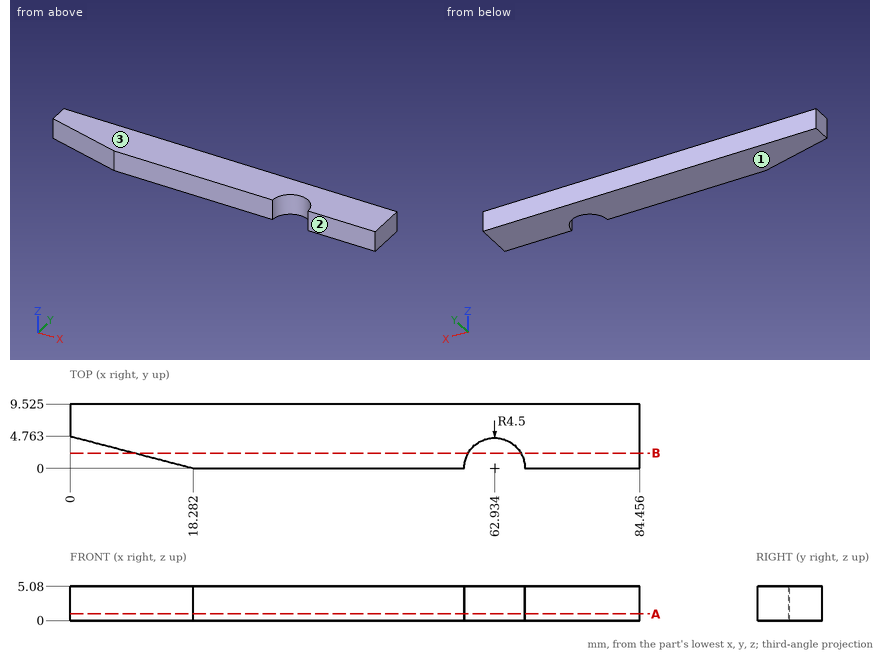
The drawing under review shows one solid part. Ordinate dimensions are in mm from its lowest x, y, z. Give positions to 0.01 mm unless a question says otherwise; leave off trailing zeros. Loops run counter-clockwise (first coordinate to the right, second up) from the corner with the lowest first, then second, coordinate; pieces in that order, holes last. Notation, with made-up numbers: M 16.25,6 L 68.25,6 A10 cw 68.25,22 Z; hole C 59.5,7.25 d7. An arc over 180 degrees is marked long. One line per question, with ' | ' between items. Start each with the question number.
1. Add section B-B (y = 2.25). Write out the cut boundary in (x, z) (1 decimal).
2. Add section A-A (z = 1). Write out the cut boundary in (x, y) (1 decimal), plus the area to 3 significant figures.
3. To check wall thickness, follow L1, parallel to Y at x = 16.5, z = 4.4 (1 decimal); L2, parallel to Y at x = 67, z = 1 (1 decimal). State the ranges of each line that lie inside material, in increasing order.
4. The part is to be moulded in two halves that separate along Z. For the marked faces 1, 2 and 3, say which applies: released by +Z, released by -Z, zero draft, split by the parting line, or undercut.
Worked out:
1) outline: M 9.6,0 L 59,0 L 59,5.1 L 9.6,5.1 Z; M 66.8,0 L 84.5,0 L 84.5,5.1 L 66.8,5.1 Z
2) outline: M 0,4.8 L 18.3,0 L 58.4,0 A4.5 cw 67.4,0 L 84.5,0 L 84.5,9.5 L 0,9.5 Z | area: 729 mm²
3) L1: y = 0.5 to 9.5 | L2: y = 1.9 to 9.5
4) face 1: released by -Z | face 2: zero draft | face 3: released by +Z
